For this review, take the finished solid that the model builds, in its own axes (mm). A direction names the side the tool comes from. Round coordinates to 2 decimals unless told otherwise and drop trailing zeros. Order: outer loops, then holes, each group sorted by start corner. A loop starts at its lowest first (then second) coordinate and runs counter-clockwise, first axis right, second up. Notation, with made-up numbers: (0, 12.25) -> (34, 12.25) arc R25 ccw to (34, 48.25) -> close; hole circle Ø3 at (77.5, -35). An arc over 180 degrees is marked (long way). Use a Markdown table: item, result. Add a question column.
1) Consider section D-D (z = 6.5). Give the number of separate pieces and of enclosed holes in the cut face, plus the area to 3 significant figures.
2) Machinability: for faces 4 (the face through (-12.5, 12.5, 0)), 5 (the face through (28, 12, 10)), which of the approach directions +Z, -Z, +X, -X, +Y, -Y give a long, thin tool a straight path to every point of the face, cutting with its end or side? Answer none if there is none.
3) Wall thickness on line 1 along Z through (x, y) = (48.5, -8.5); line 2 along Y through (x, z) = (45, 5.25); line 3 along X through (y, z) = (-30, 5): over which ranges is each line inside the solid? List them lowest first. Write a range as [from, to].
4) Draft analysis for pull direction X (two halves, no side actions). For faces 1 (the face through (-2.64, -59.94, 5.07)), 2 (the face through (23.4, 2.4, 29.7)), 3 (the face through (-40.043, -0.651, 4.93)), state which applies: pulls with the +X half, pulls with the -X half, needs draft (parallel to the pull), parting line crosses it, or undercut.
5) Clearance check with flat-ended pins moving along their axes: P1, Ø9, axis at x = -45, y = 0, coming from the +Z side; P2, Ø4, axis at y = 27.5, z = 18, coming from the +X side; P3, Ø5, axis at y = -0.5, z = 6, coming from the +X side; P4, Ø16, axis at x = 31.82, y = -31.82, coming from the +Z side. State where each tip first meets the part, or that it passes through.
6) Consider section B-B (z = 26.5). State the section outline as (x, y) points.
7) Consider section C-C (x = 45). State the section outline as (y, z) points.
8) Consider section A-A (y = 0). State the section outline as (x, z) points.
Autodesk Inventor part; units mm, degrees
ref_plane "Work Plane1" through (30, 0, 45) normal (1, 0, 0) x (0, 0, -1)
ref_plane "YZ Plane" through (0, 0, 0) normal (1, 0, 0) x (0, 1, 0)
ref_plane "XZ Plane" through (0, 0, 0) normal (0, 1, 0) x (-1, 0, 0)
sketch "Sketch2" plane through (0, 0, 0) normal (1, 0, 0) x (0, 1, 0)
  line L0 (0, 58.5) -> (0, -4.5)
  line L1 (-6, 0) -> (78, 0)
  line L2 (60, 0) -> (60, 10)
  line L3 (60, 10) -> (30, 10)
  line L4 (30, 10) -> (30, 45)
  line L5 (30, 45) -> (0, 45)
  line L6 (0, 0) -> (60, 0)
  line L7 (0, 45) -> (0, 0)
  dimension "d0" = 60
  dimension "d1" = 30
  dimension "d2" = 10
  dimension "d3" = 35
revolve "Revolution1" add sketch "Sketch2" angle 360 about axis through (0, 0, 0) along (0, 0, -1)
hole "Hole1" at (0, 0, 45) direction (0, 0, -1) diameter 35 end through all
sketch "Sketch3" plane through (0, 0, 10) normal (0, 0, 1) x (1, 0, 0)
  line L0 (-72, 0) -> (96, 0)
  line L1 (0, 96) -> (0, -72)
  point P0 (45, 0)
  dimension "d14" = 45
hole "Hole2" at (45, 0, 10) direction (0, 0, -1) diameter 10 end through all
pattern_circular "Circular Pattern1" count 8 over 360 about axis through (0, 0, -10) along (0, 0, 1) of "Hole2"
ref_plane "Work Plane1" through (30, 0, 45) normal (1, 0, 0) x (0, 0, -1)
sketch "Sketch4" plane through (30, 0, 45) normal (1, 0, 0) x (0, 0, -1)
  line L0 (-13.5, 0) -> (49.5, 0)
  line L1 (45, -72) -> (45, 96)
  line L2 (45, -60) -> (45, 60)
  line L3 (0, -30) -> (0, 30)
  point P0 (18.5, 0)
  dimension "d26" = 18.5
hole "Hole3" at (30, 0, 26.5) direction (-1, 0, 0) diameter 8 end through all
properties part number "hub"
Results list:
| question | item | result |
|---|---|---|
| 1 | separate pieces | 1 |
| 1 | enclosed holes | 9 |
| 1 | area | 9,720 mm2 |
| 2 | face 4 | -Z, +X, -X, +Y, -Y |
| 2 | face 5 | +Z |
| 3 | line 1 | [0, 10] |
| 3 | line 2 | [-39.69, -5], [5, 39.69] |
| 3 | line 3 | [-51.96, -36.48], [-27.16, 27.16], [36.48, 51.96] |
| 4 | face 1 | parting line crosses it |
| 4 | face 2 | needs draft |
| 4 | face 3 | undercut |
| 5 | P1 | through |
| 5 | P2 | x = 15.8 |
| 5 | P3 | x = 60 |
| 5 | P4 | z = 10 |
| 6 | outline | (-29.73, -4) arc R30 ccw to (29.73, -4) -> (17.04, -4) arc R17.5 cw to (-17.04, -4) -> close; (-29.73, 4) -> (-17.04, 4) arc R17.5 cw to (17.04, 4) -> (29.73, 4) arc R30 ccw to start |
| 7 | outline | (-39.69, 0) -> (-5, 0) -> (-5, 10) -> (-39.69, 10) -> close; (5, 0) -> (39.69, 0) -> (39.69, 10) -> (5, 10) -> close |
| 8 | outline | (-60, 0) -> (-50, 0) -> (-50, 10) -> (-60, 10) -> close; (-40, 0) -> (-17.5, 0) -> (-17.5, 22.5) -> (-30, 22.5) -> (-30, 10) -> (-40, 10) -> close; (-30, 30.5) -> (-17.5, 30.5) -> (-17.5, 45) -> (-30, 45) -> close; (17.5, 0) -> (40, 0) -> (40, 10) -> (30, 10) -> (30, 22.5) -> (17.5, 22.5) -> close; (17.5, 30.5) -> (30, 30.5) -> (30, 45) -> (17.5, 45) -> close; (50, 0) -> (60, 0) -> (60, 10) -> (50, 10) -> close |
